```python
from build123d import *

# Parameters (mm, degrees)
F0_W      = 26
F0_H      = 26
F0_W_2    = 16
F0_H_2    = 16
F1_DEPTH  = 2
F2_DEPTH  = 100
F3_W      = 26
F3_H      = 26
F3_W_2    = 18
F3_H_2    = 18
F4_DEPTH  = 4
F6_D      = 2.7
F6_DEPTH  = 4
F6_TIP    = 0.8111618357
F7_W      = 16
F7_H      = 96
F8_DEPTH  = 26.001
F9_W      = 16
F9_H      = 98
F10_DEPTH = 26.001


with BuildPart() as f1:
    # F0 (on Top) → F1 (new body)
    with BuildSketch(Plane.XY):
        Rectangle(F0_W, F0_H)
        Rectangle(F0_W_2, F0_H_2, mode=Mode.SUBTRACT)
        Rectangle(F0_W_2, F0_H_2)
    extrude(amount=F1_DEPTH)

    # F0 (on Top) → F2 (join)
    with BuildSketch(Plane.XY):
        Rectangle(F0_W, F0_H)
        Rectangle(F0_W_2, F0_H_2, mode=Mode.SUBTRACT)
    extrude(amount=F2_DEPTH)

    # F3 (on face) → F4 (join)
    with BuildSketch(Plane.XY.offset(100)):
        Rectangle(F3_W, F3_H)
        Rectangle(F3_W_2, F3_H_2, mode=Mode.SUBTRACT)
    extrude(amount=F4_DEPTH)

    # F6
    with Locations(Plane.XY.offset(104)):
        with Locations((-10.5, 10.5), (10.5, 10.5), (-10.5, -10.5), (10.5, -10.5)):
            Hole(F6_D / 2, depth=F6_DEPTH)
            with Locations((0, 0, -(F6_DEPTH + F6_TIP / 2))):  # 118° drill point
                Cone(0, F6_D / 2, F6_TIP, mode=Mode.SUBTRACT)

    # F7 (on face) → F8 (cut, through all)
    with BuildSketch(Plane.YZ.offset(13)):
        with Locations((0.015812546, 50)):
            Rectangle(F7_W, F7_H)
    extrude(amount=-F8_DEPTH, mode=Mode.SUBTRACT)

    # F9 (on face) → F10 (cut, through all)
    with BuildSketch(Plane(origin=(0, 13, 0), x_dir=(-1, 0, 0), z_dir=(0, 1, 0))):
        with Locations((0, 51)):
            Rectangle(F9_W, F9_H)
    extrude(amount=-F10_DEPTH, mode=Mode.SUBTRACT)


solid = f1.part
```
Design review of the part built by this model. Coordinates are the model's own, in mm. A direction names the side the tool comes from. Give positions to 0.01 mm unless a question says otherwise; leave off trailing zeros. Write each loop counter-clockwise with the first axis right and the second up, starting at its lowest first coordinate (ties: lowest second). Pieces come first, ordered by that corner, then holes. Notation, with made-up numbers: (-11.5, 87) - (4.5, 87) arc R22 ccw to (4.5, 112) - close; hole circle Ø6 at (-24.5, 10). An arc over 180 degrees is marked (long way). Return JSON: item names as keys, results as strings. Group by question number.
(1) We need section C-C, the plane z = 34. Give the boundary of the cut face in (x, y), then the cut area to 3 significant figures.
(2) Insertion check: pin 1 (3.5 mm diameter, centred on x = -10.5, y = -10.5, fed in from +Z); pin 2 (10 mm diameter, centred on x = -2.5, y = 2.5, fed in from +Z). Each pin has a flat end and moves straight along its axis. Give the tip position at first contact, or say it passes through.
(3) We need section A-A, the plane x = 7. Give the boundary of the cut face in (y, z).
(4) Machinability: for faces 1 (the flat face through (0, 0, 2)), 2 (the flat face through (-9, 0, 102)), 3 (the flat face through (-10, 0, 98)), 4 (the flat face through (0, -11, 100)), which of the approach directions +Z, -Z, +X, -X, +Y, -Y give a long, thin tool a straight path to every point of the face, cutting with its end or side? Answer none if there is none.
(5) We need section B-B, the plane y = -5.25. Give the boundary of the cut face in (x, z), then the cut area to 3 significant figures.
(6) To check wall thickness, follow probe 1 along X at (y, z) = (-10.5, 101.9); probe 2 along Z at (x, y) = (11.5, -4); probe 3 along Z at (x, y) = (-8.25, 2). State the ranges of each line that lie inside material, in increasing order.
(7) Mouldability with a two-part tool opening along Y and no side actions: class faces 5 (the flat face through (-9, -13, 51)), 6 (the flat face through (-13, -9, 51)), 7 (the flat face through (11, 0, 98)), 8 (the cylindrical face through (9.774, 11.638, 101.972)) as +Y half, -Y half, draft (parallel to the pull), parting line (faces both ways), or undercut.
Reported:
{
 "1": {"outline": "(-13, -13) - (-8, -13) - (-8, -7.98) - (-13, -7.98) - close; (-13, 8.02) - (-8, 8.02) - (-8, 13) - (-13, 13) - close; (8, -13) - (13, -13) - (13, -7.98) - (8, -7.98) - close; (8, 8.02) - (13, 8.02) - (13, 13) - (8, 13) - close", "area": "100 mm2"},
 "2": {"pin 1": "stops at z = 104", "pin 2": "stops at z = 2"},
 "3": {"outline": "(-13, 0) - (13, 0) - (13, 2) - (-13, 2) - close; (-13, 100) - (-9, 100) - (-9, 104) - (-13, 104) - close; (9, 100) - (13, 100) - (13, 104) - (9, 104) - close"},
 "4": {"face 1": "none", "face 2": "+Z", "face 3": "+X, -X", "face 4": "+Y, -Y"},
 "5": {"outline": "(-13, 0) - (13, 0) - (13, 2) - (-13, 2) - close; (-13, 98) - (-8, 98) - (-8, 100) - (-9, 100) - (-9, 104) - (-13, 104) - close; (8, 98) - (13, 98) - (13, 104) - (9, 104) - (9, 100) - (8, 100) - close", "area": "104 mm2"},
 "6": {"probe 1": "x = -13 to -11.85, -9.15 to 9.15, 11.85 to 13", "probe 2": "z = 0 to 2, 98 to 104", "probe 3": "z = 0 to 2, 98 to 100"},
 "7": {"face 5": "-Y half", "face 6": "draft", "face 7": "undercut", "face 8": "undercut"}
}
